Check sheet for the drawn part. Datum: minimum x, y, z corner. Units: mm. A direction names the side the tool comes from. Round coordinates to 2 decimals unless told otherwise and drop trailing zeros. Write each loop counter-clockwise with the first axis right and the second up, starting at its lowest first coordinate (ties: lowest second). Pieces come first, ordered by that corner, then holes. Notation, with made-up numbers: (-32.75, -35.75) -> (13.25, -35.75) arc R18 ccw to (13.25, -1.75) -> close; hole circle Ø5 at (38.25, 43). An arc over 180 degrees is marked (long way). One line per item, written item: value.
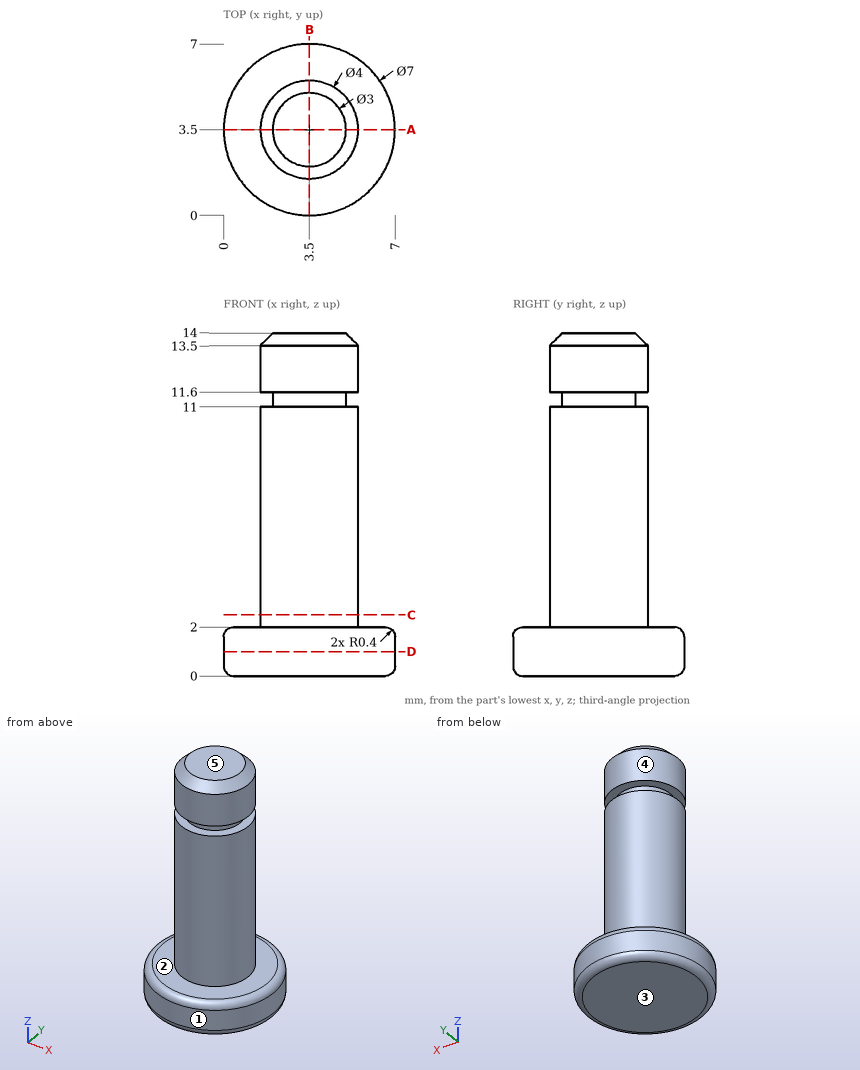
Item 1: Sectioned sample at A-A on y = 3.5. Enter the section's corners in (x, z), and give its area (3 significant figures).
Answer:
outline: (0, 0.4) arc R0.4 ccw to (0.4, 0) -> (6.6, 0) arc R0.4 ccw to (7, 0.4) -> (7, 1.6) arc R0.4 ccw to (6.6, 2) -> (5.5, 2) -> (5.5, 11) -> (5, 11) -> (5, 11.6) -> (5.5, 11.6) -> (5.5, 13.5) -> (5, 14) -> (2, 14) -> (1.5, 13.5) -> (1.5, 11.6) -> (2, 11.6) -> (2, 11) -> (1.5, 11) -> (1.5, 2) -> (0.4, 2) arc R0.4 ccw to (0, 1.6) -> close
area: 61.0 mm^2
Item 2: Tool access check on the marked faces 4 and 5. Record the directions out of +Z, -Z, +X, -X, +Y, -Y that give a thin tool (end or side, any length) a straight path to the whole face; none if there is none.
Answer:
face 4: +Z
face 5: +Z, +X, -X, +Y, -Y
Item 3: Sectioned sample at C-C on z = 2.5. Enter the section's corners in (x, y), and give its area (3 significant figures).
Answer:
outline: circle Ø4 at (3.5, 3.5)
area: 12.6 mm^2
Item 4: Thickness scan on line 1 (Z direction, x = 5, y = 0.75); line 2 (Y direction, x = 4.25, z = 8.5); line 3 (Z direction, x = 2, y = 4). Record the ranges inside material, lowest first.
Answer:
line 1: z = 0 to 2
line 2: y = 1.65 to 5.35
line 3: z = 0 to 11, 11.6 to 13.92
Item 5: Mould release check, pull along Z, two halves, no side actions. Record for the marked faces 1, 2 and 3: pulls with the +Z half, pulls with the -Z half, needs draft (parallel to the pull), parting line crosses it, or undercut.
Answer:
face 1: needs draft
face 2: pulls with the +Z half
face 3: pulls with the -Z half
Item 6: Depth check by flat-ended pin: P1, Ø1, axis at y = 1.5, z = 9, coming from the +X side; P2, Ø3, axis at x = 5, z = 4.5, coming from the +Y side; P3, Ø1.5, axis at x = 1, z = 8.5, coming from the +Y side. Enter the tip coordinate at first touch or a pass-through.
Answer:
P1: stops at x = 4.82
P2: stops at y = 5.5
P3: stops at y = 4.47
Item 7: Sectioned sample at D-D on z = 1. Enter the section's corners in (x, y).
Answer:
outline: circle Ø7 at (3.5, 3.5)
